Read the model definition and answer for the solid it produces. Units are mm, in the model's axes. A direction names the side the tool comes from. Coordinates: 2 decimals unless noted, no trailing zeros. Write each loop counter-clockwise with the first axis right and the second up, starting at its lowest first coordinate (ties: lowest second). Pieces come first, ordered by that corner, then holes.
(1) Given pin 1 (1.2 mm diameter, centred on x = -2.5, y = 1.5, fed in from -Z); pin 2 (1 mm diameter, centred on x = 3.5, z = 4.5, fed in from -Y), each flat-ended and moving along its own axis, determine where each tip first touches the part or whether it passes through.
(2) The part is cut by section C-C, the plane x = 0.5. Determine the outline of the cut face in (y, z), and give its area (3 significant figures).
(3) Determine the mould class of faces 3 (the flat face through (-0.1, 4.3, -14)), 4 (the flat face through (-7.15, 3, 0)), 5 (the flat face through (0, 4, -1)), 6 (the flat face through (5.65, 2, -1)) for opening direction X: pulls with the +X half, pulls with the -X half, needs draft (parallel to the pull), parting line crosses it, or undercut.
(4) The part is cut by section B-B, the plane z = 10.25. Determine the outline of the cut face in (x, y).
(5) Which of the six approach directions +Z, -Z, +X, -X, +Y, -Y give full straight-line access (tool end or side, diameter ignored) to faces 1 (the flat face through (-5.65, 2, -1)), 2 (the flat face through (7.15, 3, 0))?
(6) The part is cut by section A-A, the plane y = 1.25. Determine the outline of the cut face in (x, z), and give its area (3 significant figures).
(7) Straight lines are drawn through the part: line 1 along X through (y, z) = (3.85, 4.25); line 2 along Z through (x, y) = (3.75, 1.4); line 3 along Y through (x, z) = (-1, 1.5). For each, find the intervals that lie inside material, in ascending order.
```python
from build123d import *

# Parameters (mm, degrees)
BOSS_EXTRUDE1_DEPTH = 4
SKETCH2_W           = 14.3
SKETCH2_H           = 28
BOSS_EXTRUDE2_DEPTH = 2


with BuildPart() as part:
    # Sketch1 → Boss-Extrude1 (new body)
    with BuildSketch(Plane(origin=(0, 0, 0), x_dir=(1, 0, 0), z_dir=(0, 1, 0))):
        Polygon((-5.65, -12.5), (-5.65, 12.5), (-5.65, 14), (-7.15, 14), (-7.15, -14), (7.15, -14), (7.15, 14), (5.65, 14), (5.65, 12.5), (5.65, -12.5), align=None)
    extrude(amount=BOSS_EXTRUDE1_DEPTH)

    # Sketch2 → Boss-Extrude2 (add)
    with BuildSketch(Plane(origin=(0, 4, 0), x_dir=(1, 0, 0), z_dir=(0, 1, 0))):
        Rectangle(SKETCH2_W, SKETCH2_H)
    extrude(amount=BOSS_EXTRUDE2_DEPTH)


solid = part.part
```
Computed:
1. pin 1: stops at z = 12.5
1. pin 2: stops at y = 4
2. outline: (0, 12.5) - (4, 12.5) - (4, -14) - (6, -14) - (6, 14) - (0, 14) - close
2. area: 62.0 mm2
3. face 3: needs draft
3. face 4: pulls with the -X half
3. face 5: undercut
3. face 6: undercut
4. outline: (-7.15, 0) - (-5.65, 0) - (-5.65, 4) - (5.65, 4) - (5.65, 0) - (7.15, 0) - (7.15, 6) - (-7.15, 6) - close
5. face 1: -Z, -Y
5. face 2: +Z, -Z, +X, +Y, -Y
6. outline: (-7.15, -14) - (-5.65, -14) - (-5.65, 12.5) - (5.65, 12.5) - (5.65, -14) - (7.15, -14) - (7.15, 14) - (-7.15, 14) - close
6. area: 101 mm2
7. line 1: x = -7.15 to -5.65, 5.65 to 7.15
7. line 2: z = 12.5 to 14
7. line 3: y = 4 to 6
